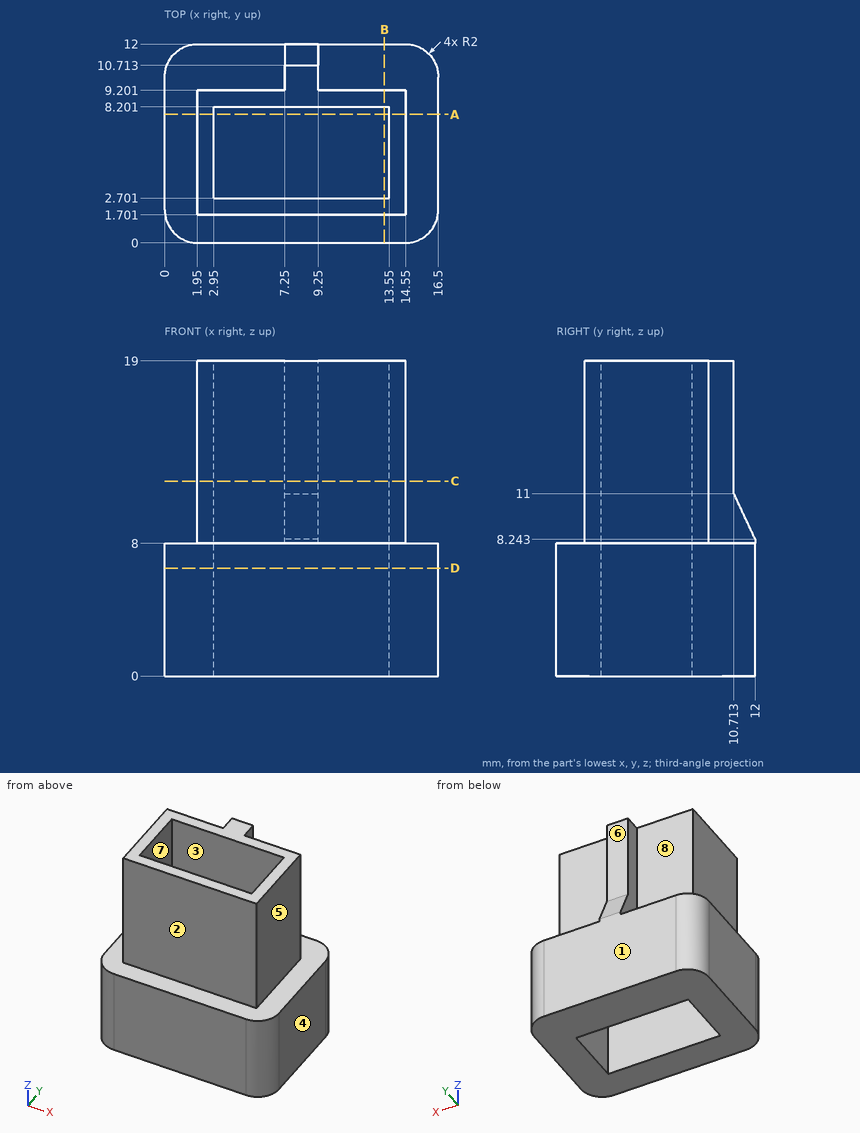
Source: three-view drawing plus pictorial views. Frame: mm from the lowest corner of the part. A direction names the side the tool comes from. Round coordinates to 2 decimals unless told otherwise and drop trailing zeros. Write each loop counter-clockwise with the first axis right and the second up, starting at its lowest first coordinate (ties: lowest second). Pieces come first, ordered by that corner, then holes. Notation, with made-up numbers: M 43,-20.75 L 58,-20.75 A20 ccw 58,13.25 Z; hole C 40.5,-9.75 d2. An arc over 180 degrees is marked long. One line per item, written item: value. Start each with the question number.
Item 1: Set-up query: the marked faces 5, 6, 7 and 8. Return all of +Z, -Z, +X, -X, +Y, -Y with unobstructed straight access to the full face (end or side cutting, diameter ignored); none if empty.
Item 2: Pin query (flat end, axial travel): pin 1 (0.8 mm diameter, centred on y = 10.5, z = 11, fed in from -X); pin 2 (1.6 mm diameter, centred on x = 12.5, z = 12.5, fed in from +Y); pin 3 (1 mm diameter, centred on y = 4.5, z = 13, fed in from -X). Return the tip coordinate at first contact, or that it passes through.
Item 3: Section query C-C (z = 11.75). Return the cut outline in (x, y).
Item 4: Section query D-D (z = 6.5). Return the cut outline in (x, y), plus the area to 3 significant figures.
Item 5: Ray query, L1, parallel to Y at x = 13, z = 12.5; L2, parallel to X at y = 5.5, z = 7.75; L3, parallel to X at y = 6.5, z = 12. Return the intervals inside material, ascending. Write a range as from..to.
Item 6: Section query B-B (x = 13.25). Return the cut outline in (y, z).
Item 7: Section query A-A (y = 7.75). Return the cut outline in (x, z).
Item 8: Mould query, pull axis Y, two halves, no side actions, for the marked faces 1, 2, 3 and 4. Classes: pulls with the +Y half, pulls with the -Y half, needs draft (parallel to the pull), parting line crosses it, or undercut.
Result set:
1. face 5: +Z, +X, +Y, -Y
1. face 6: +Z, +X, -X, +Y
1. face 7: +Z, -Z
1. face 8: +Z, -X, +Y
2. pin 1: stops at x = 7.25
2. pin 2: stops at y = 9.2
2. pin 3: stops at x = 1.95
3. outline: M 1.95,1.7 L 14.55,1.7 L 14.55,9.2 L 9.25,9.2 L 9.25,10.71 L 7.25,10.71 L 7.25,9.2 L 1.95,9.2 Z; hole M 2.95,2.7 L 13.55,2.7 L 13.55,8.2 L 2.95,8.2 Z
4. outline: M 0,2 A2 ccw 2,0 L 14.5,0 A2 ccw 16.5,2 L 16.5,10 A2 ccw 14.5,12 L 2,12 A2 ccw 0,10 Z; hole M 2.95,2.7 L 13.55,2.7 L 13.55,8.2 L 2.95,8.2 Z
4. area: 136 mm²
5. L1: y = 1.7..2.7, 8.2..9.2
5. L2: x = 0..2.95, 13.55..16.5
5. L3: x = 1.95..2.95, 13.55..14.55
6. outline: M 0,0 L 2.7,0 L 2.7,19 L 1.7,19 L 1.7,8 L 0,8 Z; M 8.2,0 L 12,0 L 12,8 L 9.2,8 L 9.2,19 L 8.2,19 Z
7. outline: M 0,0 L 2.95,0 L 2.95,19 L 1.95,19 L 1.95,8 L 0,8 Z; M 13.55,0 L 16.5,0 L 16.5,8 L 14.55,8 L 14.55,19 L 13.55,19 Z
8. face 1: pulls with the +Y half
8. face 2: pulls with the -Y half
8. face 3: undercut
8. face 4: needs draft
